Could you check a few things on this model? Use its own coordinates, in mm. Round coordinates to 2 decimals unless told otherwise and drop trailing zeros. Loops run counter-clockwise (first coordinate to the right, second up) from the corner with the lowest first, then second, coordinate; pieces in that order, holes last. Notation, with made-up numbers: M 82.5,-31 L 92.5,-31 A29 ccw 92.5,2 Z; hole C -15,-24.75 d5. An arc over 180 degrees is marked long. Answer in a Markdown table with one row per item.
```python
from build123d import *

# Parameters (mm, degrees)
SKETCH1_W           = 300
SKETCH1_H           = 150
BOSS_EXTRUDE1_DEPTH = 5
CUT_EXTRUDE1_REACH  = 7
SKETCH2_R           = 3


with BuildPart() as part:
    # Sketch1 → Boss-Extrude1 (new body)
    with BuildSketch(Plane(origin=(0, 0, 0), x_dir=(1, 0, 0), z_dir=(0, 1, 0))):
        Rectangle(SKETCH1_W, SKETCH1_H)
    extrude(amount=BOSS_EXTRUDE1_DEPTH)

    # Sketch2 → Cut-Extrude1 (cut, up to next)
    with BuildSketch(Plane(origin=(0, 5, 0), x_dir=(1, 0, 0), z_dir=(0, 1, 0)), mode=Mode.PRIVATE) as cut_extrude1_sk1:
        with Locations((-50, 0)):
            Circle(SKETCH2_R)
    cut_extrude1_tool1 = extrude(cut_extrude1_sk1.sketch, amount=-CUT_EXTRUDE1_REACH, mode=Mode.PRIVATE) & part.part
    add(cut_extrude1_tool1.solids().sort_by_distance((-50, 5, 0))[0], mode=Mode.SUBTRACT)
    # Sketch2 → Cut-Extrude1 (cut, up to next)
    with BuildSketch(Plane(origin=(0, 5, 0), x_dir=(1, 0, 0), z_dir=(0, 1, 0)), mode=Mode.PRIVATE) as cut_extrude1_sk2:
        with Locations((50, 0)):
            Circle(SKETCH2_R)
    cut_extrude1_tool2 = extrude(cut_extrude1_sk2.sketch, amount=-CUT_EXTRUDE1_REACH, mode=Mode.PRIVATE) & part.part
    add(cut_extrude1_tool2.solids().sort_by_distance((50, 5, 0))[0], mode=Mode.SUBTRACT)


solid = part.part
```
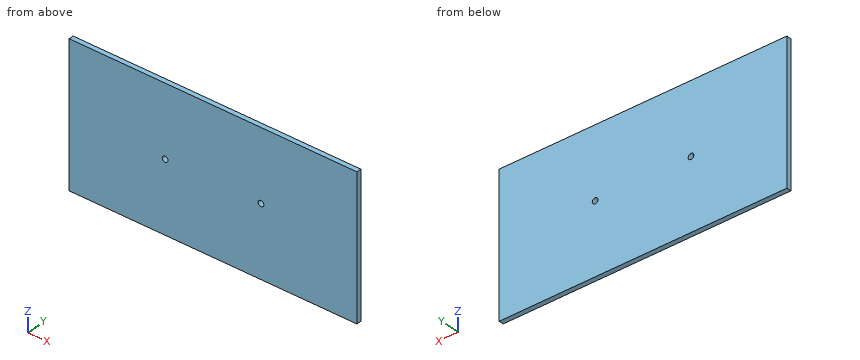
1) I want a section at A-A, the plane z = 0. Please give me the cut outline in (x, y), plus the area to 3 significant figures.
Computed:
| item | result |
|---|---|
| outline | M -150,0 L -53,0 L -53,5 L -150,5 Z; M -47,0 L 47,0 L 47,5 L -47,5 Z; M 53,0 L 150,0 L 150,5 L 53,5 Z |
| area | 1,440 mm² |
2) Will these pins go through, and if not, where does the flat tip stop? P1, Ø4, axis at x = 119, z = -20, coming from the -Y side; P2, Ø5, axis at x = -50, z = 0, coming from the +Y side.
Computed:
| item | result |
|---|---|
| P1 | stops at y = 0 |
| P2 | passes through |
3) I want a section at B-B, the plane x = -50. Please give me the cut outline in (y, z).
Computed:
| item | result |
|---|---|
| outline | M 0,-75 L 5,-75 L 5,-3 L 0,-3 Z; M 0,3 L 5,3 L 5,75 L 0,75 Z |
4) I need wall thicknesses on line 1 (X direction, y = 2.05, z = 0); line 2 (Z direction, x = -50, y = 3.75); line 3 (X direction, y = 4.35, z = 1.5). Which ranges of each line are inside material? Lowest first, please.
Computed:
| item | result |
|---|---|
| line 1 | x = -150 to -53, -47 to 47, 53 to 150 |
| line 2 | z = -75 to -3, 3 to 75 |
| line 3 | x = -150 to -52.6, -47.4 to 47.4, 52.6 to 150 |
